Source: three-view drawing plus pictorial views. Frame: mm from the lowest corner of the part. A direction names the side the tool comes from. Give positions to 0.01 mm unless a question says otherwise; leave off trailing zeros. Loops run counter-clockwise (first coordinate to the right, second up) from the corner with the lowest first, then second, coordinate; pieces in that order, holes last. Notation, with made-up numbers: M 27.5,-28.75 L 76.5,-28.75 A18 cw 76.5,-23.75 Z; hole C -19,17.25 d5. An arc over 180 degrees is marked long. Write item = value, one per line.
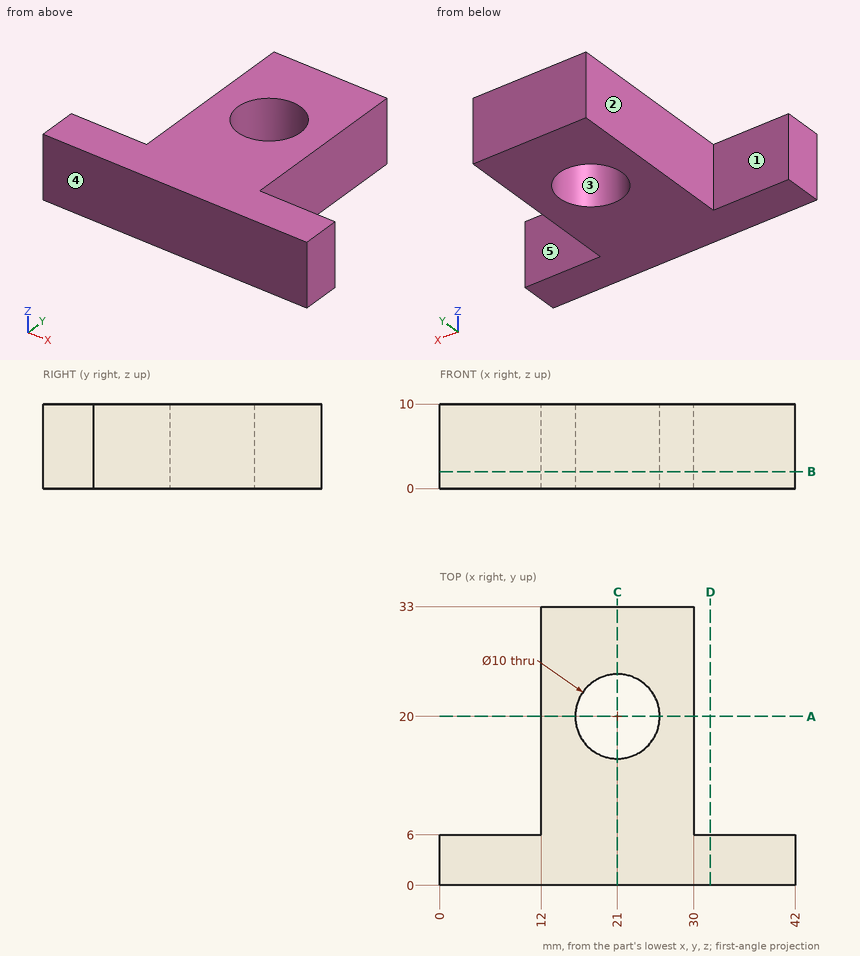
1. Cut plane B-B, the plane z = 2. Return the cut outline in (x, y).
Derived:
outline = M 0,0 L 42,0 L 42,6 L 30,6 L 30,33 L 12,33 L 12,6 L 0,6 Z; hole C 21,20 d10
2. Pull-direction query (X, two-part tool) for the marked faces 1, 2 and 3; classes: +X half, -X half, draft (parallel to the pull), parting line (faces both ways), or undercut.
Derived:
face_1 = draft
face_2 = -X half
face_3 = undercut
3. Cut plane C-C, the plane x = 21. Return the cut outline in (y, z).
Derived:
outline = M 0,0 L 15,0 L 15,10 L 0,10 Z; M 25,0 L 33,0 L 33,10 L 25,10 Z
4. Cut plane A-A, the plane y = 20. Return the cut outline in (x, z).
Derived:
outline = M 12,0 L 16,0 L 16,10 L 12,10 Z; M 26,0 L 30,0 L 30,10 L 26,10 Z
5. Cut plane D-D, the plane x = 32. Return the cut outline in (y, z), then the cut area to 3 significant figures.
Derived:
outline = M 0,0 L 6,0 L 6,10 L 0,10 Z
area = 60.0 mm²
6. First-contact query: pin 1 Ø4 at (y, z) = (11, 1.5) entering from -X; pin 2 Ø3 at (y, z) = (13, 8.5) entering from +X; pin 3 Ø5 at (x, z) = (38, 7.5) entering from +Y; pin 4 Ø6 at (x, z) = (35, 7) entering from -Y. Flat tips, straight axial feed; report the tip coordinate or a pass-through.
Derived:
pin_1 = 12
pin_2 = 30
pin_3 = 6
pin_4 = 0
7. Material intervals for probe 1 along Y at (x, z) = (21, 7.75); probe 2 along X at (y, z) = (30, 7); probe 3 along Y at (x, z) = (39.5, 8.5), sorted ascending. Write a range as from..to.
Derived:
probe_1 = 0..15, 25..33
probe_2 = 12..30
probe_3 = 0..6
8. Reachability of the marked faces 4 and 5 from +Z, -Z, +X, -X, +Y, -Y: full face, straight path, thin tool, end or side. Return the list, or none.
Derived:
face_4 = +Z, -Z, +X, -X, -Y
face_5 = +Z, -Z, +X, +Y
